from build123d import *

# Parameters (mm, degrees)
BOSS_EXTRUDE1_DEPTH     = 14
BOSS_EXTRUDE2_DEPTH     = 2
SKETCH3_W               = 0.354356076
SKETCH3_H               = 11.846889002
CUT_EXTRUDE1_DEPTH      = 3.199876682
CUT_EXTRUDE1_DEPTH_BACK = 3.199876682


with BuildPart() as part:
    # Sketch1 → Boss-Extrude1 (new body)
    with BuildSketch(Plane(origin=(0, 0, 0), x_dir=(1, 0, 0), z_dir=(0, 1, 0))):
        with BuildLine():
            Line((-1.145643924, 0.5), (-1.5, 0.5))
            Line((-1.5, 0.5), (-1.5, -0.5))
            Line((-1.5, -0.5), (-1.145643924, -0.5))
            ThreePointArc((-1.145643924, -0.5), (0, -1.25), (1.145643924, -0.5))
            Line((1.145643924, -0.5), (1.5, -0.5))
            Line((1.5, -0.5), (1.5, 0.5))
            Line((1.5, 0.5), (1.145643924, 0.5))
            ThreePointArc((1.145643924, 0.5), (0, 1.25), (-1.145643924, 0.5))
        make_face()
    extrude(amount=BOSS_EXTRUDE1_DEPTH)

    # Sketch2 → Boss-Extrude2 (add)
    with BuildSketch(Plane(origin=(0, 14, 0), x_dir=(1, 0, 0), z_dir=(0, 1, 0))):
        Polygon((-1.553767561, -1.708549004), (0.702763061, -2.199876682), (2.256530622, -0.491327678), (1.553767561, 1.708549004), (-0.702763061, 2.199876682), (-2.256530622, 0.491327678), align=None)
    extrude(amount=BOSS_EXTRUDE2_DEPTH)

    # Sketch3 → Cut-Extrude1 (cut, two sides)
    with BuildSketch(Plane.XY) as cut_extrude1_sk:
        with Locations((1.322821962, 7.070449387)):
            Rectangle(SKETCH3_W, SKETCH3_H)
        with Locations((-1.322821962, 7.070449387)):
            Rectangle(SKETCH3_W, SKETCH3_H)
    extrude(amount=CUT_EXTRUDE1_DEPTH, mode=Mode.SUBTRACT)
    extrude(cut_extrude1_sk.sketch, amount=-CUT_EXTRUDE1_DEPTH_BACK, mode=Mode.SUBTRACT)


solid = part.part
Check sheet for the modelled part. Datum: model origin and axes. Units: mm. A direction names the side the tool comes from. Give positions to 0.01 mm unless a question says otherwise; leave off trailing zeros. Order: outer loops, then holes, each group sorted by start corner. A loop starts at its lowest first (then second) coordinate and runs counter-clockwise, first axis right, second up. Notation, with made-up numbers: (-39, 14) - (-11, 14) arc R27 cw to (-11, 41) - close; hole circle Ø4 at (57.5, -20). An arc over 180 degrees is marked (long way). Answer as CSV lines item,"result".
1. Tool access check on faces 4 (the face through (1.146, 7, 0)), 5 (the face through (0.02, 6.9, -1.25)), 6 (the face through (1.5, 0.6, 0)). Record the directions out of +Z, -Z, +X, -X, +Y, -Y that give a thin tool (end or side, any length) a straight path to the whole face; none if there is none.
Result sheet:
face 4,"+Z, -Z, +X"
face 5,"-Z, -Y"
face 6,"+Z, -Z, +X, -Y"
2. Section check C-C (x = 1.7). Record the boundary of the cut face in (y, z), then the cut area to 3 significant figures.
Result sheet:
outline,"(14, -1.25) - (16, -1.25) - (16, 1.1) - (14, 1.1) - close"
area,"4.71 mm²"
3. Section check B-B (z = -0.8). Record the boundary of the cut face in (x, y), then the cut area to 3 significant figures.
Result sheet:
outline,"(-1.98, 14) - (-0.96, 14) - (-0.96, 0) - (0.96, 0) - (0.96, 14) - (1.84, 14) - (1.84, 16) - (-1.98, 16) - close"
area,"34.5 mm²"
4. Section check A-A (y = 13.5). Record the boundary of the cut face in (x, z).
Result sheet:
outline,"(-1.5, -0.5) - (-1.15, -0.5) arc R1.25 ccw to (1.15, -0.5) - (1.5, -0.5) - (1.5, 0.5) - (1.15, 0.5) arc R1.25 ccw to (-1.15, 0.5) - (-1.5, 0.5) - close"
5. Section check D-D (y = 11.5). Record the boundary of the cut face in (x, z).
Result sheet:
outline,"(-1.15, -0.5) arc R1.25 ccw to (1.15, -0.5) - (1.15, 0.5) arc R1.25 ccw to (-1.15, 0.5) - close"
6. Go/stop test with flat-tipped pins: P1, Ø0.5, axis at y = 9, z = 0, coming from the -X side; P2, Ø0.8, axis at y = 7, z = 0, coming from the +X side; P3, Ø0.8, axis at y = 0.5, z = 0, coming from the +X side; P4, Ø1.3, axis at x = 0, z = -0.5, coming from the -Y side. Record where each tip stops, or that it passes through.
Result sheet:
P1,"x = -1.15"
P2,"x = 1.15"
P3,"x = 1.5"
P4,"y = 0"
7. Scan lines: probe 1 along X at (y, z) = (0.5, -0.45); probe 2 along X at (y, z) = (8.5, -0.25); probe 3 along Y at (x, z) = (1.6, -0.15). Record each from-to range of solid material in increasing order. Write a range as from..to.
Result sheet:
probe 1,"-1.5..1.5"
probe 2,"-1.15..1.15"
probe 3,"14..16"
8. Mould release check, pull along Y, two halves, no side actions. Record for faces 1 (the face through (-1.91, 14.99, 0.59)), 2 (the face through (-1.146, 7, 0)), 3 (the face through (0, 16, 0)): released by +Y, released by -Y, zero draft, split by the parting line, or undercut.
Result sheet:
face 1,"zero draft"
face 2,"undercut"
face 3,"released by +Y"
